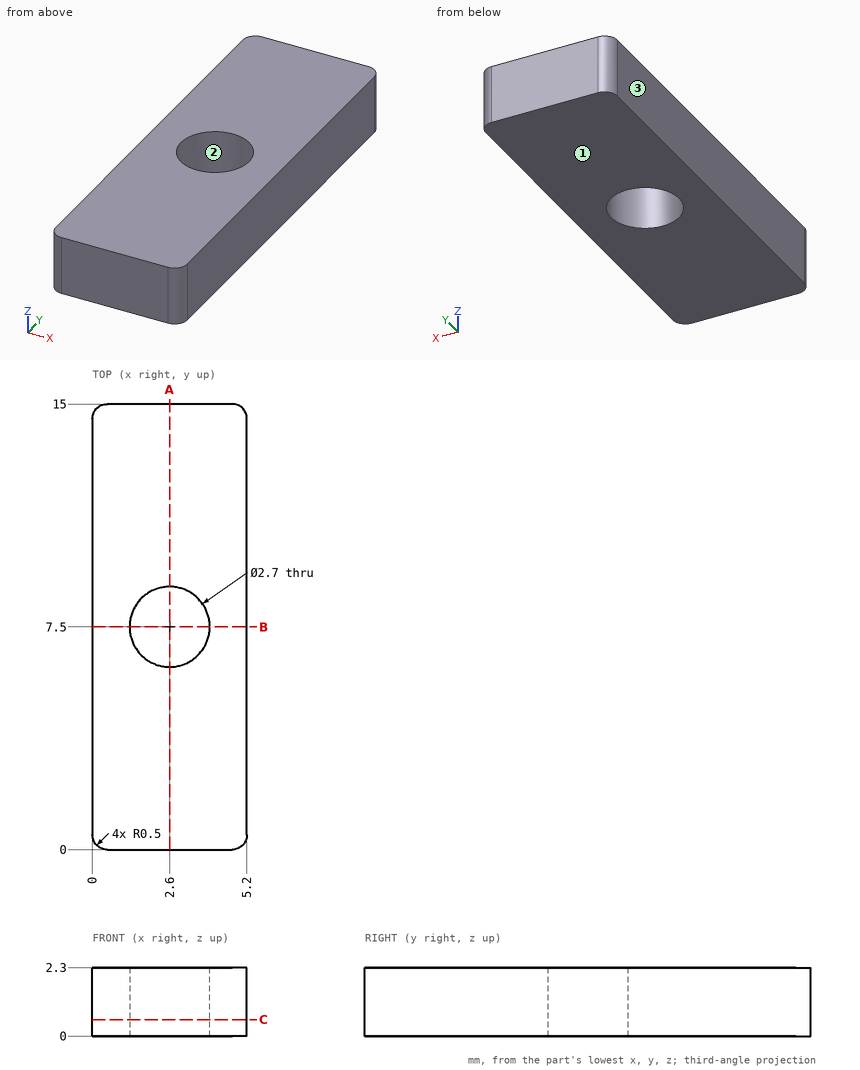
Source: three-view drawing plus pictorial views. Frame: mm from the lowest corner of the part. Coordinates: 2 decimals unless noted, no trailing zeros. Loops run counter-clockwise (first coordinate to the right, second up) from the corner with the lowest first, then second, coordinate; pieces in that order, holes last. Notation, with made-up numbers: (-2, 47.5) - (41, 47.5) arc R21 cw to (41, 86.5) - close; hole circle Ø11 at (10, 7). An arc over 180 degrees is marked (long way). One line per question, with ' | ' between items.
1) Section C-C, the plane z = 0.55. Return loops of the section in (x, y).
Report:
outline: (0, 0.5) arc R0.5 ccw to (0.5, 0) - (4.7, 0) arc R0.5 ccw to (5.2, 0.5) - (5.2, 14.5) arc R0.5 ccw to (4.7, 15) - (0.5, 15) arc R0.5 ccw to (0, 14.5) - close; hole circle Ø2.7 at (2.6, 7.5)
2) Line query: line 1 along Y through (x, z) = (2.6, 1.4); line 2 along X through (y, z) = (7.25, 0.1); line 3 along Y through (x, z) = (3.3, 1.35). Output: solid intervals per line, ascending.
Report:
line 1: y = 0 to 6.15, 8.85 to 15 | line 2: x = 0 to 1.27, 3.93 to 5.2 | line 3: y = 0 to 6.35, 8.65 to 15
3) Pull-direction query (X, two-part tool) for the marked faces 1, 2 and 3; classes: released by +X, released by -X, zero draft, split by the parting line, or undercut.
Report:
face 1: zero draft | face 2: undercut | face 3: released by -X
4) Section A-A, the plane x = 2.6. Return loops of the section in (y, z).
Report:
outline: (0, 0) - (6.15, 0) - (6.15, 2.3) - (0, 2.3) - close; (8.85, 0) - (15, 0) - (15, 2.3) - (8.85, 2.3) - close
5) Section B-B, the plane y = 7.5. Return loops of the section in (x, z), then the cut area to 3 significant figures.
Report:
outline: (0, 0) - (1.25, 0) - (1.25, 2.3) - (0, 2.3) - close; (3.95, 0) - (5.2, 0) - (5.2, 2.3) - (3.95, 2.3) - close | area: 5.75 mm²
